Could you check a few things on this model? Use its own coordinates, in mm. A direction names the side the tool comes from. Give positions to 0.01 mm unless a question says otherwise; leave off trailing zeros. Loops run counter-clockwise (first coordinate to the right, second up) from the corner with the lowest first, then second, coordinate; pieces in that order, holes last. Notation, with made-up numbers: (83, -4) -> (138, -4) arc R14 cw to (138, 1) -> close; hole circle Ø10 at (46.25, 8). An arc over 180 degrees is marked (long way). Write item = value, one per line. Start each with the question number.
1) I want a section at B-B (x = 10.16). List the corners of the cut face in (y, z) for me (1 decimal).
2) I want a section at C-C (z = 0). List the corners of the cut face in (x, y) for me (1 decimal).
3) I need wall thicknesses on probe 1 along X at (y, z) = (-2.5, 5.5) (3 decimals); probe 2 along Y at (x, z) = (1.65, 0); probe 3 along Z at (x, y) = (1.9, 0). Which ranges of each line are inside material? Lowest first, please. Write a range as from..to.
4) I want a section at D-D (y = -16). List the corners of the cut face in (x, z) for me.
5) I want a section at A-A (y = -6). List the corners of the cut face in (x, z) for me (1 decimal).
6) If we mould it in two halves opening along Z, with no side actions, what happens to faces 3 (the face through (17.145, -3.5, 0.1)), 4 (the face through (8.91, -16.17, 3.08)), 5 (the face through (10, -15, -7.938))? For each: +Z half, -Z half, draft (parallel to the pull), parting line (faces both ways), or undercut.
7) On a 3-axis mill with a long thin cutter (end or side, diameter ignored), from which of +Z, -Z, +X, -X, +Y, -Y can I reach the whole of each face in a straight line? I mean faces 1 (the face through (1.565, -3.186, 0.708)), 2 (the face through (3.175, -3.5, 0.1)). Say none if no direction works.
8) I'm going to push flat-ended pins straight in: pin 1 Ø2 at (x, y) = (14.5, -3) entering from -Z; pin 2 Ø6 at (x, y) = (11, -12.5) entering from -Z. Where does each tip first touch, or does it pass through?
from build123d import *

# Parameters (mm, degrees)
SKETCH2_R           = 7.9375
SKETCH2_R_2         = 3.2639
BOSS_EXTRUDE1_DEPTH = 20.32
SKETCH3_W           = 13.97
SKETCH3_H           = 25.4
CUT_EXTRUDE1_DEPTH  = 12.7
SKETCH4_R           = 3.2639
CUT_EXTRUDE2_DEPTH  = 29.143111169


with BuildPart() as part:
    # Sketch2 → Boss-Extrude1 (new body)
    # profile 1 of 2: a face of its own
    with BuildSketch(Plane(origin=(0, 0, 0), x_dir=(0, 0, -1), z_dir=(1, 0, 0))):
        with BuildLine():
            ThreePointArc((7.9375, 0), (0, -7.9375), (-7.9375, 0))
            Line((-7.9375, 0), (-7.9375, -17.78))
            Line((-7.9375, -17.78), (7.9375, -17.78))
            Line((7.9375, -17.78), (7.9375, 0))
        make_face()
    # profile 2 of 2: a face of its own
    with BuildSketch(Plane(origin=(0, 0, 0), x_dir=(0, 0, -1), z_dir=(1, 0, 0))):
        Circle(SKETCH2_R)
        Circle(SKETCH2_R_2, mode=Mode.SUBTRACT)
    extrude(amount=BOSS_EXTRUDE1_DEPTH)

    # Sketch3 → Cut-Extrude1 (cut, symmetric)
    with BuildSketch(Plane.XY):
        with Locations((10.16, -1.905)):
            Rectangle(SKETCH3_W, SKETCH3_H)
    extrude(amount=CUT_EXTRUDE1_DEPTH, both=True, mode=Mode.SUBTRACT)

    # Sketch4 → Cut-Extrude2 (cut, through all)
    with BuildSketch(Plane(origin=(0, 0, 0), x_dir=(1, 0, 0), z_dir=(0, 1, 0))):
        with Locations(Location((10.16, -0.0635, 0), (0, 0, 270))):
            Circle(SKETCH4_R)
    extrude(amount=-CUT_EXTRUDE2_DEPTH, mode=Mode.SUBTRACT)


solid = part.part
Answer list:
q1.outline = (-17.8, -7.9) -> (-14.6, -7.9) -> (-14.6, -3.2) -> (-17.8, -3.2) -> close; (-17.8, 3.3) -> (-14.6, 3.3) -> (-14.6, 7.9) -> (-17.8, 7.9) -> close
q2.outline = (0, -17.8) -> (6.9, -17.8) -> (6.9, -14.6) -> (3.2, -14.6) -> (3.2, -3.3) -> (0, -3.3) -> close; (0, 3.3) -> (3.2, 3.3) -> (3.2, 7.9) -> (0, 7.9) -> close; (13.4, -17.8) -> (20.3, -17.8) -> (20.3, -3.3) -> (17.1, -3.3) -> (17.1, -14.6) -> (13.4, -14.6) -> close; (17.1, 3.3) -> (20.3, 3.3) -> (20.3, 7.9) -> (17.1, 7.9) -> close
q3.probe_1 = 0..3.175, 17.145..20.32
q3.probe_2 = -17.78..-3.26, 3.26..7.94
q3.probe_3 = -7.94..-3.26, 3.26..7.94
q4.outline = (0, -7.94) -> (20.32, -7.94) -> (20.32, 7.94) -> (0, 7.94) -> close; hole circle Ø6.53 at (10.16, 0.06)
q5.outline = (0, -7.9) -> (3.2, -7.9) -> (3.2, 7.9) -> (0, 7.9) -> close; (17.1, -7.9) -> (20.3, -7.9) -> (20.3, 7.9) -> (17.1, 7.9) -> close
q6.face_3 = draft
q6.face_4 = undercut
q6.face_5 = -Z half
q7.face_1 = +X, -X
q7.face_2 = +Z, -Z, +Y
q8.pin_1 = through
q8.pin_2 = -7.94
